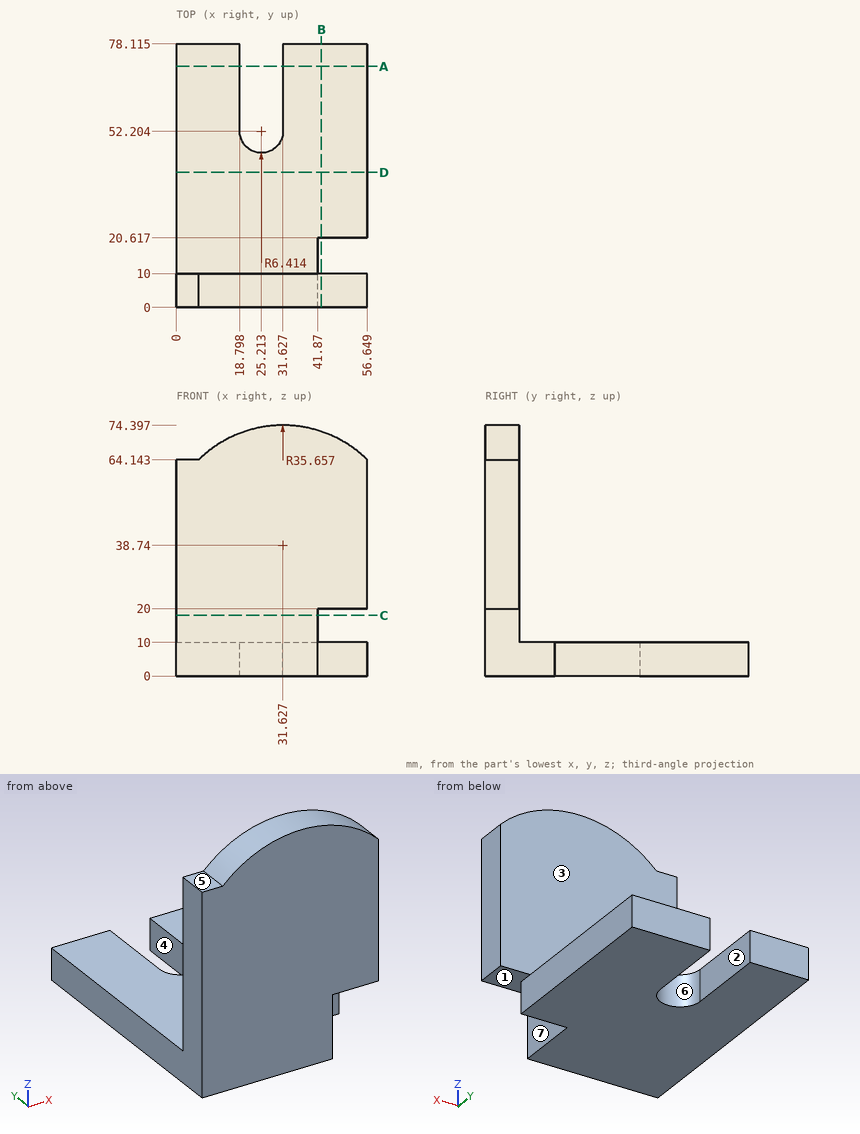
For this review, use the dimensioned drawing (mm, ordinates from the lowest corner) and the shaded views. A direction names the side the tool comes from. Give positions to 0.01 mm unless a question says otherwise; leave off trailing zeros. Order: outer loops, then holes, each group sorted by start corner. A loop starts at its lowest first (then second) coordinate and runs counter-clockwise, first axis right, second up. Notation, with made-up numbers: (-36, -39) - (-4, -39) arc R20 ccw to (-4, -20) - close; hole circle Ø1 at (38, 63). An arc over 180 degrees is marked (long way). Use a Markdown table: item, result. Add a question column.
(1) Clearance check with flat-ended pins moving along their axes: P1, Ø1.5, axis at x = 46, z = 66.5, coming from the +Y side; P2, Ø11, axis at x = 50.5, y = 3, coming from the -Z side; P3, Ø7.5, axis at x = 4, y = 3.5, coming from the +Z side. State where each tip first meets the part, or that it passes through.
(2) Add section D-D on y = 40. Give the boundary of the cut face in (x, z).
(3) Add section B-B on x = 43. Give the boundary of the cut face in (y, z) (1 decimal), then the cut area to 3 significant figures.
(4) Add section A-A on y = 71.5. Give the boundary of the cut face in (x, z).
(5) Mouldability with a two-part tool opening along X and no side actions: class the marked faces 4, 5, 6 and 7 as +X half, -X half, draft (parallel to the pull), parting line (faces both ways), or undercut.
(6) Wall thickness on probe 1 along Y at (x, z) = (25.5, 53); probe 2 along X at (y, z) = (10.5, 4): over which ranges is each line inside the solid? List them lowest first. Write a range as [from, to].
(7) Machinability: for the marked faces 1, 2 and 3, which of the approach directions +Z, -Z, +X, -X, +Y, -Y give a long, thin tool a straight path to every point of the face, cutting with its end or side? Answer none if there is none.
(8) Add section C-C on z = 18. Give the boundary of the cut face in (x, y).
Report:
| question | item | result |
|---|---|---|
| 1 | P1 | stops at y = 10 |
| 1 | P2 | stops at z = 20 |
| 1 | P3 | stops at z = 65.22 |
| 2 | outline | (0, 0) - (56.65, 0) - (56.65, 10) - (0, 10) - close |
| 3 | outline | (0, 20) - (10, 20) - (10, 72.5) - (0, 72.5) - close; (20.6, 0) - (78.1, 0) - (78.1, 10) - (20.6, 10) - close |
| 3 | area | 1,100 mm² |
| 4 | outline | (0, 0) - (18.8, 0) - (18.8, 10) - (0, 10) - close; (31.63, 0) - (56.65, 0) - (56.65, 10) - (31.63, 10) - close |
| 5 | face 4 | undercut |
| 5 | face 5 | draft |
| 5 | face 6 | undercut |
| 5 | face 7 | +X half |
| 6 | probe 1 | y = [0, 10] |
| 6 | probe 2 | x = [0, 41.87] |
| 7 | face 1 | -Z, +X, +Y, -Y |
| 7 | face 2 | +Z, -Z, +Y |
| 7 | face 3 | +Z, +X, -X, +Y |
| 8 | outline | (0, 0) - (41.87, 0) - (41.87, 10) - (0, 10) - close |
